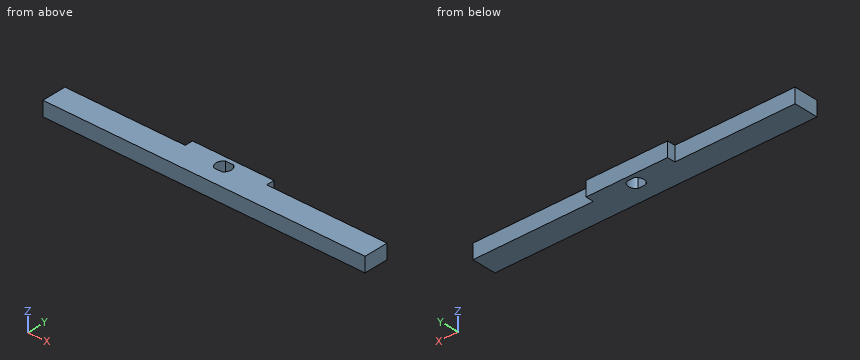
```python
from build123d import *

# Parameters (mm, degrees)
PAD_DEPTH    = 18
POCKET_DEPTH = 18


with BuildPart() as part:
    # Sketch → Pad (new body)
    with BuildSketch(Plane.XY):
        Polygon((0, 0), (-197.5, 0), (-197.5, 30), (-50, 30), (-50, 40), (0, 40), align=None)
    pad = extrude(amount=PAD_DEPTH)

    # Mirrored: Pad across Sketch V_Axis
    add(pad.mirror(Plane(origin=(0, 0, 0), x_dir=(0, 0, 1), z_dir=(1, 0, 0))))

    # Sketch001 (on DatumPlane) → Pocket (cut)
    with BuildSketch(Plane.XY.offset(18)):
        with BuildLine():
            ThreePointArc((-4.907138, 34.9), (-9.3, 27), (-4.907138, 19.1))
            Line((-4.907138, 19.1), (4.907138, 19.1))
            ThreePointArc((4.907138, 19.1), (9.3, 27), (4.907138, 34.9))
            Line((-4.907138, 34.9), (4.907138, 34.9))
        make_face()
    extrude(amount=-POCKET_DEPTH, mode=Mode.SUBTRACT)


solid = part.part
```
Geometry check sheet. Reference: the model listing, model coordinates, mm. Coordinates: 2 decimals unless noted, no trailing zeros. Order: outer loops, then holes, each group sorted by start corner. A loop starts at its lowest first (then second) coordinate and runs counter-clockwise, first axis right, second up. Notation, with made-up numbers: (62, -6) - (99, -6) arc R32 ccw to (99, 28) - close; hole circle Ø3 at (68, 55). An arc over 180 degrees is marked (long way). Answer in a Markdown table with one row per item. Add a question column.
1. Gauge pin test, flat ends, axial feed: pin 1 Ø6 at (x, z) = (-137, 4.5) entering from -Y; pin 2 Ø2 at (x, z) = (-142.5, 2.5) entering from +Y; pin 3 Ø3 at (y, z) = (36.5, 10.5) entering from -X; pin 4 Ø8 at (y, z) = (36, 12.5) entering from +X. Record the tip position at first contact, or that the pin passes through.
2. Section check B-B (y = 26.5). Enter the section's corners in (x, z).
3. Section check A-A (z = 12). Enter the section's corners in (x, y).
4. Section check C-C (x = 160). Enter the section's corners in (y, z).
5. Material ranges on L1, parallel to Y at x = -88, z = 12.75; L2, parallel to X at y = 28.5, z = 10.5; L3, parallel to X at y = 25, z = 15, recorded low to high. Write a range as [from, to].
Data:
| question | item | result |
|---|---|---|
| 1 | pin 1 | stops at y = 0 |
| 1 | pin 2 | stops at y = 30 |
| 1 | pin 3 | stops at x = -50 |
| 1 | pin 4 | stops at x = 50 |
| 2 | outline | (-197.5, 0) - (-9.29, 0) - (-9.29, 18) - (-197.5, 18) - close; (9.29, 0) - (197.5, 0) - (197.5, 18) - (9.29, 18) - close |
| 3 | outline | (-197.5, 0) - (197.5, 0) - (197.5, 30) - (50, 30) - (50, 40) - (-50, 40) - (-50, 30) - (-197.5, 30) - close; hole (-4.91, 19.1) - (4.91, 19.1) arc R9.3 ccw to (4.91, 34.9) - (-4.91, 34.9) arc R9.3 ccw to start |
| 4 | outline | (0, 0) - (30, 0) - (30, 18) - (0, 18) - close |
| 5 | L1 | y = [0, 30] |
| 5 | L2 | x = [-197.5, -9.18], [9.18, 197.5] |
| 5 | L3 | x = [-197.5, -9.08], [9.08, 197.5] |
